from build123d import *

# Parameters (mm, degrees)
F0_W     = 27.270341292
F0_H     = 11.066971153
F1_DEPTH = 10
F3_DEPTH = 49.001


with BuildPart() as f1:
    # F0 (on Top) → F1 (new body)
    with BuildSketch(Plane.XY):
        with BuildLine():
            ThreePointArc((-17, 0), (0, 17), (17, 0))
            Line((17, 0), (17, 29))
            Line((17, 29), (27, 29))
            Line((27, 29), (27, 32))
            Line((27, 32), (17, 32))
            Line((17, 32), (-17, 32))
            Line((-17, 32), (-27, 32))
            Line((-27, 32), (-27, 29))
            Line((-27, 29), (-17, 29))
            Line((-17, 29), (-17, 0))
        make_face()
        with Locations((0, 23.4665144235)):
            Rectangle(F0_W, F0_H, mode=Mode.SUBTRACT)
        with BuildLine():
            Line((17, 0), (15, 0))
            ThreePointArc((15, 0), (0, -15), (-15, 0))
            Line((-15, 0), (-17, 0))
            ThreePointArc((-17, 0), (0, -17), (17, 0))
        make_face()
        with BuildLine():
            ThreePointArc((-15, 0), (0, 15), (15, 0))
            Line((15, 0), (17, 0))
            ThreePointArc((17, 0), (0, 17), (-17, 0))
            Line((-17, 0), (-15, 0))
        make_face()
    extrude(amount=F1_DEPTH)

    # F2 (on face) → F3 (cut, through all)
    with BuildSketch(Plane(origin=(0, 32, 0), x_dir=(-1, 0, 0), z_dir=(0, 1, 0))):
        with BuildLine():
            Line((-26.1, 5), (-22.9, 5))
            ThreePointArc((-22.9, 5), (-24.5, 6.6), (-26.1, 5))
        make_face()
        with BuildLine():
            ThreePointArc((-26.1, 5), (-24.5, 3.4), (-22.9, 5))
            Line((-22.9, 5), (-26.1, 5))
        make_face()
        with BuildLine():
            Line((22.9, 5), (26.1, 5))
            ThreePointArc((26.1, 5), (24.5, 6.6), (22.9, 5))
        make_face()
        with BuildLine():
            ThreePointArc((22.9, 5), (24.5, 3.4), (26.1, 5))
            Line((26.1, 5), (22.9, 5))
        make_face()
    extrude(amount=-F3_DEPTH, mode=Mode.SUBTRACT)


solid = f1.part
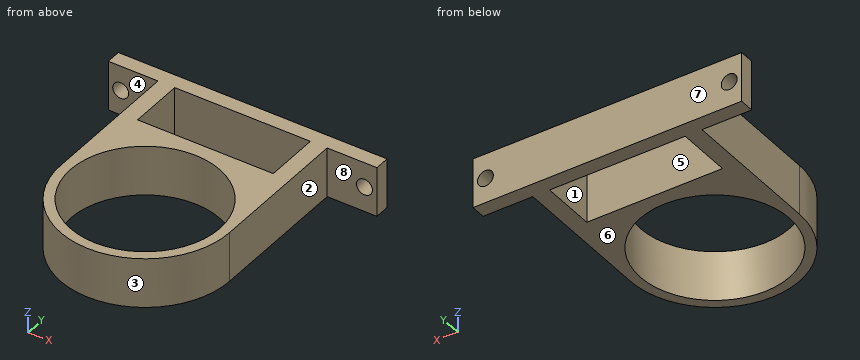
Could you check a few things on this model? Use its own coordinates, in mm. Face numbers are marked on the shaded views. A direction names the side the tool comes from. Coordinates: 2 decimals unless noted, no trailing zeros. Order: outer loops, then holes, each group sorted by start corner. A loop starts at its lowest first (then second) coordinate and runs counter-clockwise, first axis right, second up. Notation, with made-up numbers: (-10, -27.75) -> (19, -27.75) arc R23 ccw to (19, -7.75) -> close; hole circle Ø7 at (-26.75, 88). An arc over 180 degrees is marked (long way). One line per item, written item: value. Start each with the question number.
1) Imagine slicing it at A-A on x = -24.5. List the corners of the cut face in (y, z) for me.
2) If I drill on L1, parallel to X at y = 31.3, z = 5; L2, parallel to Y at x = 0, z = 3.25; L3, parallel to X at y = 20, z = 5.5, over which ranges is the centre line in solid material (lowest first)? Write a range as [from, to].
3) We'd pull the mould along Y, two halves only. Please class the marked faces 5, 6, 7 and 8: +Y half, -Y half, draft (parallel to the pull), parting line (faces both ways), or undercut.
4) Which directions (+Z, -Z, +X, -X, +Y, -Y) give clear straight access to the entire face, cutting with the end or side of a thin tool? Please do the marked faces 1, 2, 3 and 4.
5) Imagine slicing it at C-C on y = 24.5. List the corners of the cut face in (x, z) for me.
6) Imagine slicing it at D-D on x = 0. List the corners of the cut face in (y, z) for me, plus the area to 3 significant figures.
7) Imagine slicing it at B-B on z = 5. List the corners of the cut face in (x, y) for me.
8) I'm going to push flat-ended pins straight in: pin 1 (1.5 mm diameter, centred on x = -9.5, z = 8, fed in from -Y); pin 2 (1.9 mm diameter, centred on x = -24.5, z = 5, fed in from +Y); pin 3 (5 mm diameter, centred on x = 21.5, z = 4, fed in from -Y); pin 4 (3 mm diameter, centred on y = 21.5, z = 3.5, fed in from -X). Where does each tip first touch, or does it pass through?
Answer list:
1. outline: (29, 0) -> (32, 0) -> (32, 3.4) -> (29, 3.4) -> close; (29, 6.6) -> (32, 6.6) -> (32, 10) -> (29, 10) -> close
2. L1: x = [-27, -26.1], [-22.9, 22.9], [26.1, 27]
2. L2: y = [-17, -15], [15, 17.93], [29, 32]
2. L3: x = [-17, -13.64], [13.64, 17]
3. face 5: undercut
3. face 6: draft
3. face 7: +Y half
3. face 8: -Y half
4. face 1: +Z, -Z
4. face 2: +Z, -Z, +X, -Y
4. face 3: +Z, -Z, -Y
4. face 4: +Z, -Z, -X, -Y
5. outline: (-17, 0) -> (-13.64, 0) -> (-13.64, 10) -> (-17, 10) -> close; (13.64, 0) -> (17, 0) -> (17, 10) -> (13.64, 10) -> close
6. outline: (-17, 0) -> (-15, 0) -> (-15, 10) -> (-17, 10) -> close; (15, 0) -> (17.93, 0) -> (17.93, 10) -> (15, 10) -> close; (29, 0) -> (32, 0) -> (32, 10) -> (29, 10) -> close
6. area: 79.3 mm2
7. outline: (-27, 29) -> (-26.1, 29) -> (-26.1, 32) -> (-27, 32) -> close; (-22.9, 29) -> (-17, 29) -> (-17, 0) arc R17 ccw to (17, 0) -> (17, 29) -> (22.9, 29) -> (22.9, 32) -> (-22.9, 32) -> close; (26.1, 29) -> (27, 29) -> (27, 32) -> (26.1, 32) -> close; hole circle Ø30 at (0, 0); hole (-13.64, 17.93) -> (13.64, 17.93) -> (13.64, 29) -> (-13.64, 29) -> close
8. pin 1: stops at y = -14.58
8. pin 2: passes through
8. pin 3: stops at y = 29
8. pin 4: stops at x = -17
